```python
from build123d import *
from build123d.topology import SkipClean

# Parameters (mm, degrees)
BOSS_EXTRU_1_DEPTH      = 10
ESQUISSE5_R             = 10.2
ENL_V_MAT_EXTRU_1_DEPTH = 1
CONG_2_R                = 3
ESQUISSE7_W             = 2.4
ESQUISSE7_H             = 12
ENL_V_MAT_EXTRU_2_DEPTH = 8


with BuildPart() as part:
    # Esquisse1 → Boss.-Extru.1 (new body)
    with BuildSketch(Plane.XY):
        with BuildLine():
            ThreePointArc((0.614016819, 2.936491673), (1.070466269, 2.802517077), (1.5, 2.598076211))
            ThreePointArc((1.5, 2.598076211), (1.891817848, 2.328309522), (2.236067977, 2))
            Line((2.236067977, 2), (11.832159566, 2))
            ThreePointArc((11.832159566, 2), (12, 0), (11.832159566, -2))
            Line((11.832159566, -2), (2.236067977, -2))
            ThreePointArc((2.236067977, -2), (1.891817848, -2.328309522), (1.5, -2.598076211))
            ThreePointArc((1.5, -2.598076211), (1.070466269, -2.802517077), (0.614016819, -2.936491673))
            Line((0.614016819, -2.936491673), (-4.184028976, -11.246950766))
            ThreePointArc((-4.184028976, -11.246950766), (-6, -10.392304845), (-7.648130591, -9.246950766))
            Line((-7.648130591, -9.246950766), (-2.850084796, -0.936491673))
            ThreePointArc((-2.850084796, -0.936491673), (-2.962284118, -0.474207555), (-3, 0))
            ThreePointArc((-3, 0), (-2.962284118, 0.474207555), (-2.850084796, 0.936491673))
            Line((-2.850084796, 0.936491673), (-7.648130591, 9.246950766))
            ThreePointArc((-7.648130591, 9.246950766), (-6, 10.392304845), (-4.184028976, 11.246950766))
            Line((-4.184028976, 11.246950766), (0.614016819, 2.936491673))
        make_face()
    extrude(amount=BOSS_EXTRU_1_DEPTH)

    # Esquisse4 → Révolution1 (revolve)
    with SkipClean():  # the faces are left unmerged after this step: merging them gives an invalid solid
        with BuildSketch(Plane(origin=(0, 0, 0), x_dir=(1, 0, 0), z_dir=(0, 1, 0)), mode=Mode.PRIVATE) as r_volution1_sk:
            Polygon((3, -10), (0, -10), (0, 0), (12, 0), (12, -2), align=None)
        revolve(r_volution1_sk.sketch.rotate(Axis((0, 0, 10), (0, 0, -1)), 129.594068227), axis=Axis((0, 0, 10), (0, 0, -1)))

    # Esquisse5 → Enlèv. mat.-Extru.1 (cut)
    with SkipClean():  # the faces are left unmerged after this step: merging them gives an invalid solid
        with BuildSketch(Plane(origin=(0, 0, 0), x_dir=(-1, 0, 0), z_dir=(0, 0, -1))):
            Circle(ESQUISSE5_R)
        extrude(amount=-ENL_V_MAT_EXTRU_1_DEPTH, mode=Mode.SUBTRACT)

    # Esquisse6 → Enlèvement de matière-Révolution1 (revolve, cut)
    with BuildSketch(Plane(origin=(0, 0, 0), x_dir=(1, 0, 0), z_dir=(0, 1, 0)), mode=Mode.PRIVATE) as enl_vement_de_mati_re_r_volution1_sk:
        Polygon((11, 0), (15.480754368, 0), (15.480754368, -10), (7.75, -10), (7.4, -10), (7.4, -8), (8.4, -8), (11, -2), align=None)
    revolve(enl_vement_de_mati_re_r_volution1_sk.sketch.rotate(Axis((0, 0, 0), (0, 0, 1)), 180), axis=Axis((0, 0, 0), (0, 0, 1)), mode=Mode.SUBTRACT)

    # Congé2
    cong_2_edges = [part.edges().sort_by_distance(p)[0] for p in [
        (5.186746988, -8.983709309, 3.445783133),
        (-9.443834359, -4.292245317, 3.445783133),
        (5.186746988, 8.983709309, 3.445783133),
        (11, 0, 2),
    ]]
    fillet(cong_2_edges, radius=CONG_2_R)

    # Esquisse7 → Enlèv. mat.-Extru.2 (cut)
    with BuildSketch(Plane.XY.offset(10)):
        with Locations((2.2, 0)):
            Rectangle(ESQUISSE7_W, ESQUISSE7_H)
    extrude(amount=-ENL_V_MAT_EXTRU_2_DEPTH, mode=Mode.SUBTRACT)


solid = part.part
```
Part model, mm, in its own coordinate system. A direction names the side the tool comes from. Round coordinates to 2 decimals unless told otherwise and drop trailing zeros. Answer in a Markdown table with one row per item. Add a question column.
Q1. Wall check: L1, parallel to Y at x = 0, z = 0.25; L2, parallel to Z at x = 1.5, y = 2.75; L3, parallel to Z at x = -5.5, y = -2.25. Give the ranges that are in metal, low to high. Write a range as from..to.
Q2. Pin check, flat tips, straight feed: pin 1 (2.5 mm diameter, centred on y = 1, z = 6.5, fed in from +X); pin 2 (2.5 mm diameter, centred on y = 0.5, z = 5, fed in from -X); pin 3 (4 mm diameter, centred on x = -4.5, z = 1.5, fed in from +Y); pin 4 (12 mm diameter, centred on x = -8.5, y = 1.5, fed in from +Z). Stop position of each tip, or through.
Q3. 3-axis set-ups, long thin cutter, end or side, ignore diameter. For faces 5 (the face through (2, 0, 2)), 6 (the face through (-4, 7, 8)), 7 (the face through (6.6, 2, 7.7)), 8 (the face through (7, -2, 7)): which of +Z, -Z, +X, -X, +Y, -Y reach the whole face in a straight line?
Q4. Mould opens along X. For faces 1 (the face through (-4.59, -7.21, 7.66)), 2 (the face through (2, -6, 5)), 3 (the face through (-4, -7, 8)), 4 (the face through (7.4, 0, 9)) say: +X half, -X half, draft (parallel to the pull), parting line (faces both ways), or undercut.
Established:
| question | item | result |
|---|---|---|
| 1 | L1 | y = -11..-10.2, 10.2..11 |
| 1 | L2 | z = 1..2 |
| 1 | L3 | z = 1..7.38 |
| 2 | pin 1 | stops at x = 9.55 |
| 2 | pin 2 | stops at x = -10.01 |
| 2 | pin 3 | stops at y = 10.71 |
| 2 | pin 4 | stops at z = 10 |
| 3 | face 5 | +Z |
| 3 | face 6 | +Z, -X, +Y |
| 3 | face 7 | +Z, +X, +Y |
| 3 | face 8 | +Z, +X, -Y |
| 4 | face 1 | parting line |
| 4 | face 2 | undercut |
| 4 | face 3 | draft |
| 4 | face 4 | +X half |
